Check sheet for the modelled part. Datum: model origin and axes. Units: mm. Face numbers are marked on the shaded views. A direction names the side the tool comes from. Coordinates: 2 decimals unless noted, no trailing zeros. Write each loop counter-clockwise with the first axis right and the second up, starting at its lowest first coordinate (ties: lowest second). Pieces come first, ordered by that corner, then holes. Notation, with made-up numbers: M 87.25,61.25 L 116.25,61.25 A24 cw 116.25,90.25 Z; hole C 77.5,1.25 d7. An arc over 180 degrees is marked long. Answer as CSV lines item,"result". Start each with the question number.
1) Material ranges on L1, parallel to X at y = 0.95, z = -21.5; L2, parallel to Z at x = 12, y = 21.5; L3, parallel to Y at x = 0, z = -0.55, recorded low to high. Write a range as [from, to].
2) Section check C-C (y = 11.5). Record the cut outline in (x, z).
3) Access from +Z, -Z, +X, -X, +Y, -Y to the whole of each face (thin tool, end or side, straight path). Record for the marked faces 1 and 2.
4) Section check A-A (z = -7.5). Record the cut outline in (x, y), and give its area (3 significant figures).
5) Section check D-D (x = -23). Record the cut outline in (y, z).
6) Section check B-B (x = 13.75). Record the cut outline in (y, z).
7) Go/stop test with a flat-tipped pin: pin 1 Ø1 at (x, z) = (-19, -10.5) entering from +Y. Record where the tip stops, or that it passes through.
from build123d import *

# Parameters (mm, degrees)
BASE_FLANGE1_DEPTH           = 2
EDGE_FLANGE1_STRIP_W         = 12
EDGE_FLANGE1_STRIP_H         = 2
EDGE_FLANGE1_STRIP_CUT_DEPTH = 90
EDGE_FLANGE1_DEPTH           = 90
SKETCH11_R                   = 4
CUT_EXTRUDE1_DEPTH           = 69.044103345
M3X0_5_TAPPED_HOLE1_D        = 3
SKETCH14_R                   = 4
CUT_EXTRUDE2_DEPTH           = 67.828137786
M3X0_5_TAPPED_HOLE2_D        = 3


# Sheet-metal steps are written as plain solids
with BuildPart() as part:
    # Sketch1 → Base-Flange1 (new body)
    with BuildSketch(Plane.XY):
        with BuildLine():
            Line((-45, 0), (45, 0))
            Line((45, 0), (45, 37))
            ThreePointArc((45, 37), (43.535533906, 40.535533906), (40, 42))
            Line((40, 42), (-40, 42))
            ThreePointArc((-40, 42), (-43.535533906, 40.535533906), (-45, 37))
            Line((-45, 37), (-45, 0))
        make_face()
    extrude(amount=-BASE_FLANGE1_DEPTH)

    # Edge-Flange1 strip (across the edge) → Edge-Flange1 strip cut (cut)
    with BuildSketch(Plane(origin=(45, 0, -2), x_dir=(0, 1, 0), z_dir=(-1, 0, 0))):
        with Locations((-2, -1)):
            Rectangle(EDGE_FLANGE1_STRIP_W, EDGE_FLANGE1_STRIP_H)
    extrude(amount=EDGE_FLANGE1_STRIP_CUT_DEPTH, mode=Mode.SUBTRACT)

    # Edge-Flange1 section (across the edge) → Edge-Flange1 (add)
    with BuildSketch(Plane(origin=(45, 0, -2), x_dir=(0, 1, 0), z_dir=(-1, 0, 0))):
        with BuildLine():
            Line((0, 2), (0, 12.5))
            Line((0, 12.5), (2, 12.5))
            Line((2, 12.5), (2, 2))
            ThreePointArc((2, 2), (2.585786438, 0.585786438), (4, 0))
            Line((4, 0), (4, -2))
            ThreePointArc((4, -2), (1.171572875, -0.828427125), (0, 2))
        make_face()
    extrude(amount=EDGE_FLANGE1_DEPTH)

    # Mirror1: part across plane


with BuildPart() as part_1:
    add(part.part)
    add(part.part.mirror(Plane(origin=(45, 0, -14.5), x_dir=(1, 0, 0), z_dir=(0, 0, 1))))

    # Sketch11 → Cut-Extrude1 (cut, through all)
    with BuildSketch(Plane.XY):
        with Locations((-34.75, 30.8)):
            Circle(SKETCH11_R)
        with Locations((0, 30.8)):
            Circle(SKETCH11_R)
        with Locations((34.75, 30.8)):
            Circle(SKETCH11_R)
    extrude(amount=-CUT_EXTRUDE1_DEPTH, mode=Mode.SUBTRACT)

    # M3x0.5 Tapped Hole1 (through all)
    with Locations(Plane.XY):
        with Locations((-34.75, 37.8), (-34.75, 23.8), (-27.75, 30.8), (-41.75, 30.8), (0, 37.8), (0, 23.8), (-7, 30.8), (7, 30.8), (34.75, 37.8), (34.75, 23.8), (41.75, 30.8), (27.75, 30.8), (-13.75, 37.8), (13.75, 37.8)):
            Hole(M3X0_5_TAPPED_HOLE1_D / 2)

    # Sketch14 → Cut-Extrude2 (cut, through all)
    with BuildSketch(Plane(origin=(0, 2, 0), x_dir=(1, 0, 0), z_dir=(0, 1, 0))):
        with Locations(Location((-34.75, 14.5, 0), (0, 0, 270))):
            Circle(SKETCH14_R)
        with Locations(Location((0, 14.5, 0), (0, 0, 270))):
            Circle(SKETCH14_R)
        with Locations(Location((34.75, 14.5, 0), (0, 0, 270))):
            Circle(SKETCH14_R)
    extrude(amount=-CUT_EXTRUDE2_DEPTH, mode=Mode.SUBTRACT)

    # M3x0.5 Tapped Hole2 (through all)
    with Locations(Plane(origin=(0, 2, 0), x_dir=(1, 0, 0), z_dir=(0, 1, 0))):
        with Locations((-34.75, 21.5), (-34.75, 7.5), (-41.75, 14.5), (-27.75, 14.5), (0, 21.5), (0, 7.5), (-7, 14.5), (7, 14.5), (34.75, 21.5), (34.75, 7.5), (41.75, 14.5), (27.75, 14.5)):
            Hole(M3X0_5_TAPPED_HOLE2_D / 2)


solid = part_1.part
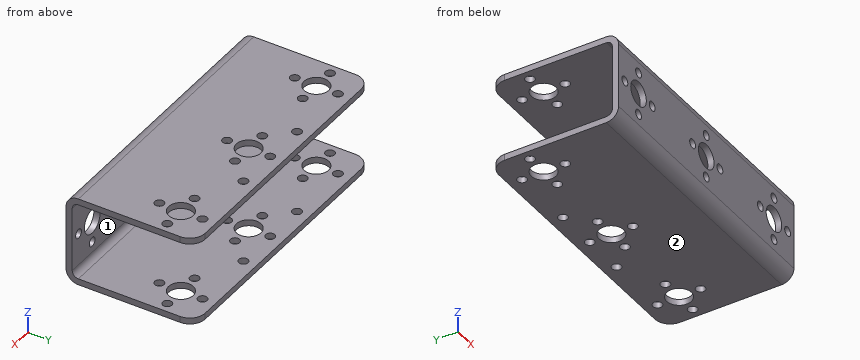
Results found:
1,L1,"x = [-45, -36.25], [-33.25, -1.5], [1.5, 33.25], [36.25, 45]"
1,L2,"z = [-29, -27], [-2, 0]"
1,L3,"y = [1.98, 22.3], [25.3, 26.8], [34.8, 36.3], [39.3, 42]"
2,outline,"M -45,-29 L 45,-29 L 45,-27 L -45,-27 Z; M -45,-2 L 45,-2 L 45,0 L -45,0 Z"
3,face 1,"+X, -X, +Y"
3,face 2,"-Z, +X, -X, +Y, -Y"
4,outline,"M -45,0 L -36.25,0 L -36.25,2 L -45,2 Z; M -33.25,0 L -1.5,0 L -1.5,2 L -33.25,2 Z; M 1.5,0 L 33.25,0 L 33.25,2 L 1.5,2 Z; M 36.25,0 L 45,0 L 45,2 L 36.25,2 Z"
4,area,"162 mm2"
5,outline,"M 0,-25 A4 ccw 4,-29 L 42,-29 L 42,-27 L 4,-27 A2 cw 2,-25 L 2,-4 A2 cw 4,-2 L 42,-2 L 42,0 L 4,0 A4 ccw 0,-4 Z"
6,outline,"M 0,-25 A4 ccw 4,-29 L 36.3,-29 L 36.3,-27 L 4,-27 A2 cw 2,-25 L 2,-4 A2 cw 4,-2 L 36.3,-2 L 36.3,0 L 4,0 A4 ccw 0,-4 Z; M 39.3,-29 L 42,-29 L 42,-27 L 39.3,-27 Z; M 39.3,-2 L 42,-2 L 42,0 L 39.3,0 Z"
7,pin 1,"stops at y = 2"
